Check sheet for the drawn part. Datum: minimum x, y, z corner. Units: mm. A direction names the side the tool comes from. Round coordinates to 2 decimals unless told otherwise and drop trailing zeros. Write each loop counter-clockwise with the first axis right and the second up, starting at its lowest first coordinate (ties: lowest second). Pieces come first, ordered by that corner, then holes. Notation, with made-up numbers: (60.5, -32.5) - (111.5, -32.5) arc R28 ccw to (111.5, 3.5) - close; hole circle Ø9 at (0, -30.5). An arc over 180 degrees is marked (long way). Answer as a JSON object with one key per item and string values.
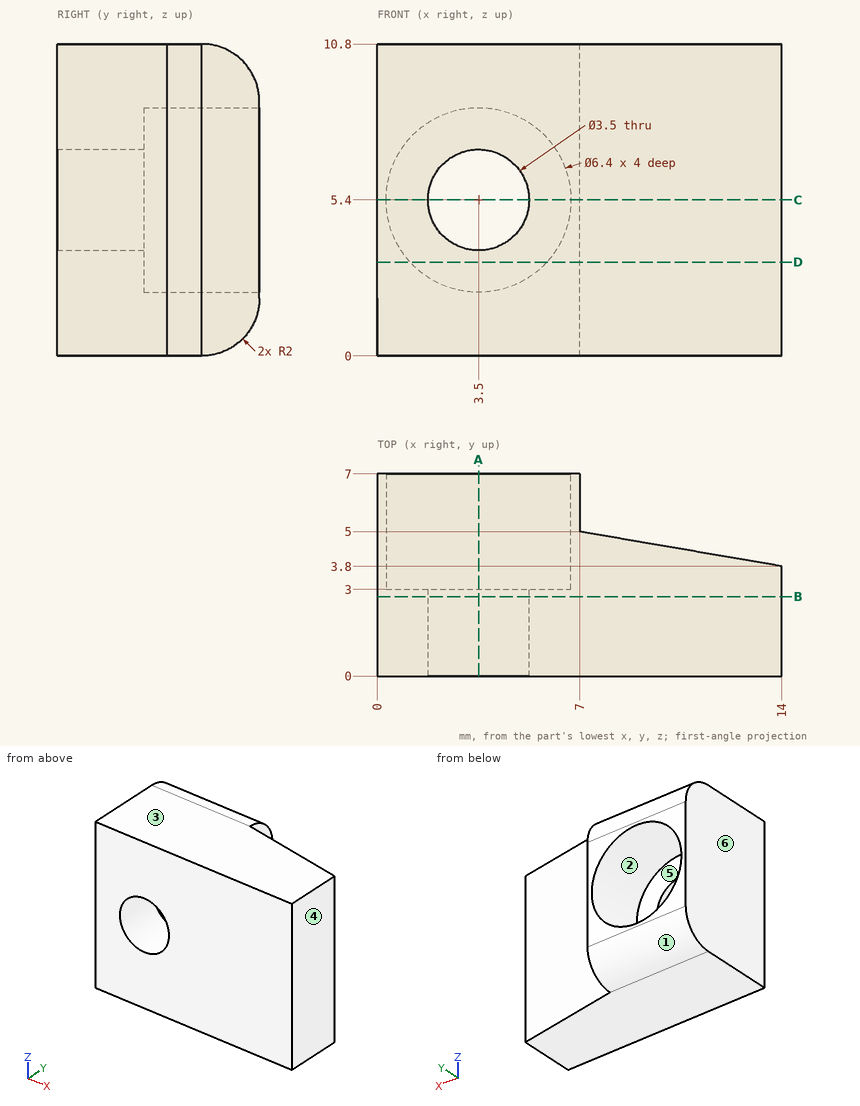
1. Cross-section at B-B (y = 2.75). Record the boundary of the cut face in (x, z).
Completed:
{"outline": "(0, 0) - (14, 0) - (14, 10.8) - (0, 10.8) - close; hole circle Ø3.5 at (3.5, 5.4)"}
2. Cross-section at A-A (x = 3.5). Record the boundary of the cut face in (y, z), plus the area to 3 significant figures.
Completed:
{"outline": "(0, 0) - (5, 0) arc R2 ccw to (7, 2) - (7, 2.2) - (3, 2.2) - (3, 3.65) - (0, 3.65) - close; (0, 7.15) - (3, 7.15) - (3, 8.6) - (7, 8.6) - (7, 8.8) arc R2 ccw to (5, 10.8) - (0, 10.8) - close", "area": "37.8 mm^2"}
3. Mould release check, pull along X, two halves, no side actions. Record for the marked faces 3, 4, 5 and 6: released by +X, released by -X, zero draft, split by the parting line, or undercut.
Completed:
{"face 3": "zero draft", "face 4": "released by +X", "face 5": "undercut", "face 6": "released by -X"}
4. Cross-section at C-C (z = 5.4). Record the boundary of the cut face in (x, y).
Completed:
{"outline": "(0, 0) - (1.75, 0) - (1.75, 3) - (0.3, 3) - (0.3, 7) - (0, 7) - close; (5.25, 0) - (14, 0) - (14, 3.8) - (7, 5) - (7, 7) - (6.7, 7) - (6.7, 3) - (5.25, 3) - close"}
5. Cross-section at D-D (z = 3.25). Record the boundary of the cut face in (x, y).
Completed:
{"outline": "(0, 0) - (14, 0) - (14, 3.8) - (7, 5) - (7, 7) - (5.87, 7) - (5.87, 3) - (1.13, 3) - (1.13, 7) - (0, 7) - close"}
6. Access from +Z, -Z, +X, -X, +Y, -Y to the whole of each face (thin tool, end or side, straight path). Record for the marked faces 1 and 2.
Completed:
{"face 1": "-Z, +X, -X, +Y", "face 2": "+Y"}
7. Material ranges on probe 1 along Z at (x, y) = (3.5, 2.05); probe 2 along X at (y, z) = (5.75, 9.75); probe 3 along Z at (x, y) = (3.5, 4.4), recorded low to high. Write a range as from..to.
Completed:
{"probe 1": "z = 0..3.65, 7.15..10.8", "probe 2": "x = 0..7", "probe 3": "z = 0..2.2, 8.6..10.8"}
